Job drawing, mm, ordinate dimensions from the low corner. One solid piece. Give positions to 0.01 mm unless a question says otherwise; leave off trailing zeros. Order: outer loops, then holes, each group sorted by start corner. A loop starts at its lowest first (then second) coordinate and runs counter-clockwise, first axis right, second up. Notation, with made-up numbers: (-25, 16) -> (16, 16) arc R18 ccw to (16, 28) -> close; hole circle Ø10 at (77, -15.75). An arc over 180 degrees is marked (long way). Write item = value, one per line. Start each with the question number.
(1) Two-plate mould, pull along Y, no slides. Class the marked faces 1, 2, 3 and 4: pulls with the +Y half, pulls with the -Y half, needs draft (parallel to the pull), parting line crosses it, or undercut.
(2) Saw through at A-A, the plane y = 11.5. List the corners of the cut face in (x, z), then the cut area to 3 significant figures.
(3) Probe line 1 along X through (y, z) = (6, 3.3); line 2 along Y through (x, z) = (20, 3.15); line 3 along X through (y, z) = (10.25, 4.25) (1 decimal). List the from-to ranges inside material, lowest first. Write a range as from..to.
(4) Flat gauge pins, fed straight in: pin 1 (1.5 mm diameter, centred on x = 23.5, y = 8, fed in from +Z); pin 2 (0.7 mm diameter, centred on x = 11.5, z = 4, fed in from -Y); pin 3 (1 mm diameter, centred on y = 4.5, z = 3, fed in from -X). Where does each tip first touch, or does it go through?
(5) Saw through at D-D, the plane x = 11. List the corners of the cut face in (y, z), then the cut area to 3 significant figures.
(6) Saw through at B-B, the plane z = 1.65. List the corners of the cut face in (x, y) (1 decimal), then the cut area to 3 significant figures.
(7) Saw through at C-C, the plane z = 5.6. List the corners of the cut face in (x, y) (1 decimal), then the cut area to 3 significant figures.
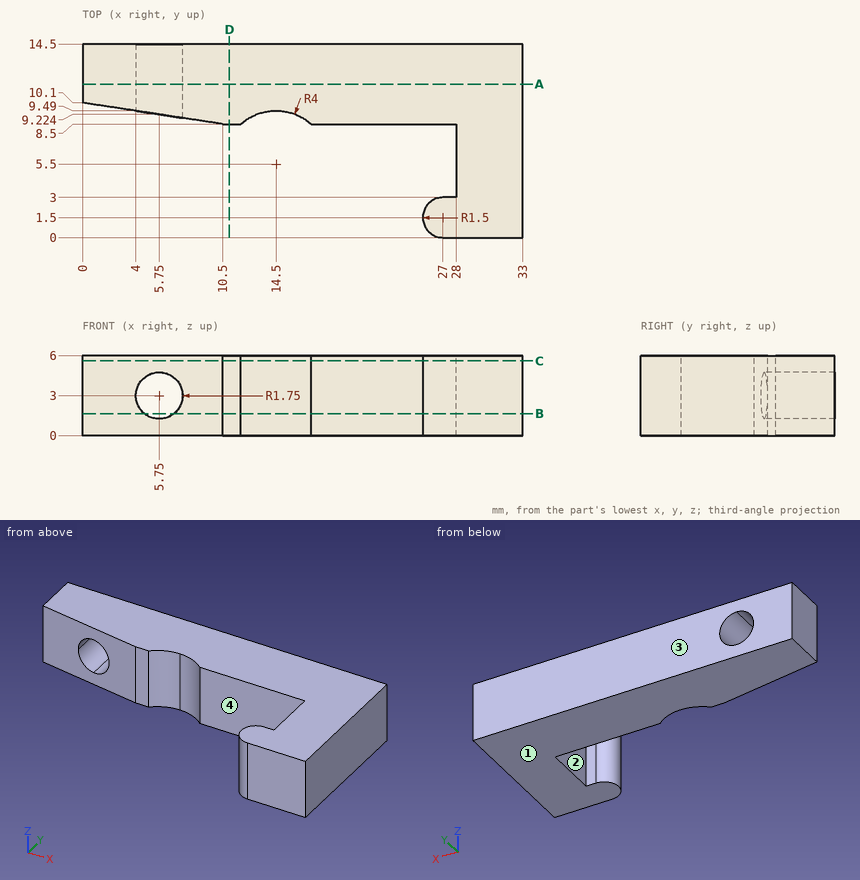
Results list:
q1.face_1 = needs draft
q1.face_2 = undercut
q1.face_3 = pulls with the +Y half
q1.face_4 = undercut
q2.outline = (0, 0) -> (33, 0) -> (33, 6) -> (0, 6) -> close; hole circle Ø3.5 at (5.75, 3)
q2.area = 188 mm^2
q3.line_1 = 28..33
q3.line_2 = 8.5..14.5
q3.line_3 = 0..4.5, 7..33
q4.pin_1 = 6
q4.pin_2 = 8.5
q4.pin_3 = 28
q5.outline = (8.5, 0) -> (14.5, 0) -> (14.5, 6) -> (8.5, 6) -> close
q5.area = 36.0 mm^2
q6.outline = (0, 10.1) -> (4.6, 9.4) -> (4.6, 14.5) -> (0, 14.5) -> close; (6.9, 9.1) -> (10.5, 8.5) -> (11.9, 8.5) arc R4 cw to (17.1, 8.5) -> (28, 8.5) -> (28, 3) -> (27, 3) arc R1.5 ccw to (27, 0) -> (33, 0) -> (33, 14.5) -> (6.9, 14.5) -> close
q6.area = 223 mm^2
q7.outline = (0, 10.1) -> (10.5, 8.5) -> (11.9, 8.5) arc R4 cw to (17.1, 8.5) -> (28, 8.5) -> (28, 3) -> (27, 3) arc R1.5 ccw to (27, 0) -> (33, 0) -> (33, 14.5) -> (0, 14.5) -> close
q7.area = 235 mm^2
